```python
from build123d import *

# Parameters (mm, degrees)
F0_W     = 184
F0_H     = 184
F0_R     = 1.5
F0_W_2   = 8
F0_H_2   = 8
F1_DEPTH = 10


with BuildPart() as f1:
    # F0 (on Top) → F1 (new body)
    with BuildSketch(Plane.XY):
        Polygon((100, 92), (92, 92), (92, 100), (-100, 100), (-100, -100), (100, -100), align=None)
        Rectangle(F0_W, F0_H, mode=Mode.SUBTRACT)
        Rectangle(F0_W, F0_H)
        with Locations((-80, -80)):
            Circle(F0_R, mode=Mode.SUBTRACT)
        with Locations((80, -80)):
            Circle(F0_R, mode=Mode.SUBTRACT)
        with Locations((-80, 80)):
            Circle(F0_R, mode=Mode.SUBTRACT)
        with Locations((80, 80)):
            Circle(F0_R, mode=Mode.SUBTRACT)
        Polygon((100, 100), (100, 92), (108, 100), (108, 108), (100, 108), (92, 100), align=None)
        with Locations((96, 96)):
            Rectangle(F0_W_2, F0_H_2)
    extrude(amount=F1_DEPTH)


solid = f1.part
```
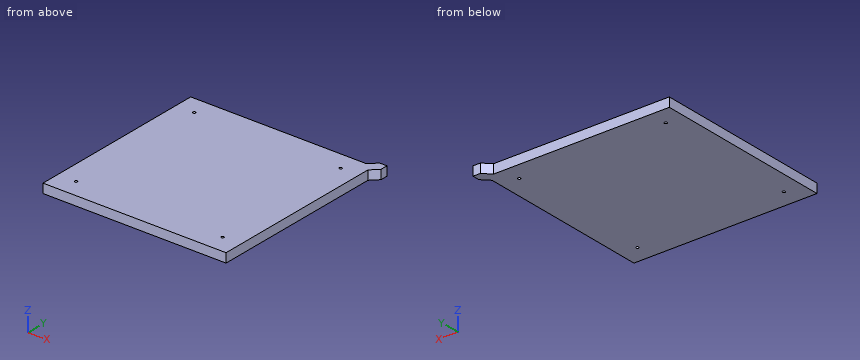
CAD build for the part. Positions are in the model's coordinates, mm. Round coordinates to 2 decimals unless told otherwise and drop trailing zeros. Write each loop counter-clockwise with the first axis right and the second up, starting at its lowest first coordinate (ties: lowest second). Pieces come first, ordered by that corner, then holes. Notation, with made-up numbers: (61, -13) - (83, -13) arc R20 ccw to (83, -7) - close; hole circle Ø9 at (78.5, 28). An arc over 180 degrees is marked (long way). Return JSON: item names as keys, results as strings. Group by question number.
Item 1: Flat gauge pins, fed straight in: pin 1 Ø5 at (x, z) = (73, 1) entering from +Y; pin 2 Ø3 at (x, y) = (-46, 26) entering from -Z; pin 3 Ø3 at (y, z) = (-43.5, 2.5) entering from +X. Where does each tip first touch, or does it go through?
Item 2: Probe probe 1 along X at (y, z) = (80, 7); probe 2 along Y at (x, z) = (-79, 5.75). List the from-to ranges inside material, lowest first.
Item 3: Band-saw the part on A-A on z = 5.75. List the corners of the cut face in (x, y), plus the area to 3 significant figures.
Item 4: Band-saw the part on B-B on y = -34. List the corners of the cut face in (x, z).
Resolved:
{
 "1": {"pin 1": "stops at y = 100", "pin 2": "stops at z = 0", "pin 3": "stops at x = 100"},
 "2": {"probe 1": "x = -100 to -81.5, -78.5 to 78.5, 81.5 to 100", "probe 2": "y = -100 to -81.12, -78.88 to 78.88, 81.12 to 100"},
 "3": {"outline": "(-100, -100) - (100, -100) - (100, 92) - (108, 100) - (108, 108) - (100, 108) - (92, 100) - (-100, 100) - close; hole circle Ø3 at (-80, -80); hole circle Ø3 at (-80, 80); hole circle Ø3 at (80, -80); hole circle Ø3 at (80, 80)", "area": "40,100 mm²"},
 "4": {"outline": "(-100, 0) - (100, 0) - (100, 10) - (-100, 10) - close"}
}
